Input: part model. Units: mm. Frame: model coordinates. A direction names the side the tool comes from. Give positions to 0.01 mm unless a question says otherwise; leave off trailing zeros. Write each loop counter-clockwise with the first axis right and the second up, starting at its lowest first coordinate (ties: lowest second). Pieces come first, ordered by that corner, then holes. Notation, with made-up numbers: (25.25, -21.5) - (47.25, -21.5) arc R29 cw to (47.25, 6.5) - close; hole circle Ø4 at (-34.5, 67). An arc over 180 degrees is marked (long way). Answer as CSV lines item,"result". Start each with the question number.
from build123d import *

# Parameters (mm, degrees)
CYLINDER001_W     = 10
CYLINDER001_H     = 10
CYLINDER001_ANGLE = 45
ARRAY_COUNT       = 8
CYLINDER_R        = 12
CYLINDER_DEPTH    = 10


with BuildPart() as array:
    # Cylinder001 → Cylinder001 (revolve)
    with BuildSketch(Plane(origin=(1, 0, 0), x_dir=(1, 0, 0), z_dir=(0, -1, 0))):
        with Locations((5, 5)):
            Rectangle(CYLINDER001_W, CYLINDER001_H)
    revolve(axis=Axis((1, 0, 0), (0, 0, 1)), revolution_arc=CYLINDER001_ANGLE)

    # Array: Array ×8 about axis
    array_axis = Axis((0, 0, 0), (0, 0, 1))


with BuildPart() as array_1:
    add(array.part)
    for i in range(1, ARRAY_COUNT):
        add(array.part.rotate(array_axis, i * 360 / ARRAY_COUNT))


with BuildPart() as array_2:
    # Array placement: moved
    add(array_1.part.moved(Location((0, 0, 1))))


with BuildPart() as cut:
    # Cylinder → Cylinder (new body)
    with BuildSketch(Plane.XY):
        Circle(CYLINDER_R)
    extrude(amount=CYLINDER_DEPTH)

    # Cut: cut Array
    add(array_2.part, mode=Mode.SUBTRACT)


solid = cut.part
1) Cut plane A-A on z = 4. State how many separate pieces and enclosed holes the cut face has, and give its area (3 significant figures).
2) Pull-direction query (X, two-part tool) for faces 3 (the flat face through (0, 0, 10)), 4 (the flat face through (-4, 4, 6)); classes: +X half, -X half, draft (parallel to the pull), parting line (faces both ways), or undercut.
3) Contact query for flat-ended pins moving along their axis: P1, Ø1, axis at y = -4, z = 6, coming from the +X side; P2, Ø2, axis at x = 8.5, y = 4.5, coming from the +Z side; P3, Ø5, axis at y = 3, z = 3, coming from the -X side. Output: stop coordinate, or through.
4) Cut plane C-C on x = 5.5. Output: boundary loops of the cut face in (y, z).
5) Material intervals for line 1 (X direction, y = 3, z = 4.5); line 2 (Y direction, x = -9.75, z = 2.5); line 3 (Y direction, x = 9.5, z = 9.5), sorted ascending. Write a range as from..to.
6) Cut plane B-B on y = 3. Output: boundary loops of the cut face in (x, z).
7) Reachability of faces 1 (the flat face through (0, 0, 0)), 2 (the flat face through (4, 3, 6)) from +Z, -Z, +X, -X, +Y, -Y: full face, straight path, thin tool, end or side. Return the list, or none.
Numbers:
1,separate pieces,"1"
1,enclosed holes,"8"
1,area,"138 mm²"
2,face 3,"draft"
2,face 4,"undercut"
3,P1,"stops at x = 11.48"
3,P2,"stops at z = 1"
3,P3,"stops at x = -11.99"
4,outline,"(-10.67, 0) - (10.67, 0) - (10.67, 10) - (9.48, 10) - (9.48, 1) - (5.5, 1) - (5.5, 10) - (4.5, 10) - (4.5, 1) - (0, 1) - (0, 10) - (-0.71, 10) - (-0.71, 1) - (-5.5, 1) - (-5.5, 10) - (-6.5, 10) - (-6.5, 1) - (-9.35, 1) - (-9.35, 10) - (-10.67, 10) - close"
5,line 1,"x = -11.62..-10.44, -3..-2, 0..0.71, 3..4, 10.54..11.62"
5,line 2,"y = -7..-4.84, 0..0.71, 4.98..7"
5,line 3,"y = -7.33..-5.47, -0.71..0, 5.27..7.33"
6,outline,"(-11.62, 0) - (11.62, 0) - (11.62, 10) - (10.54, 10) - (10.54, 1) - (4, 1) - (4, 10) - (3, 10) - (3, 1) - (0.71, 1) - (0.71, 10) - (0, 10) - (0, 1) - (-2, 1) - (-2, 10) - (-3, 10) - (-3, 1) - (-10.44, 1) - (-10.44, 10) - (-11.62, 10) - close"
7,face 1,"-Z, +X, -X, +Y, -Y"
7,face 2,"+Z"
